```python
from build123d import *

# Parameters (mm, degrees)
SKETCH2_W           = 50
SKETCH2_H           = 52
BOSS_EXTRUDE1_DEPTH = 52
SKETCH3_W           = 50
SKETCH3_H           = 50
CUT_EXTRUDE1_DEPTH  = 50
CUT_EXTRUDE3_DEPTH  = 50
SKETCH5_R           = 2
CUT_EXTRUDE4_DEPTH  = 50
SKETCH7_W           = 52
SKETCH7_H           = 2
BOSS_EXTRUDE2_DEPTH = 5
SKETCH8_R           = 2.5
CUT_EXTRUDE6_DEPTH  = 5
SKETCH10_W          = 1
SKETCH10_H          = 2
CUT_EXTRUDE7_DEPTH  = 160
SKETCH11_W          = 48
SKETCH11_H          = 2
BOSS_EXTRUDE3_DEPTH = 3
SKETCH12_W          = 48
SKETCH12_H          = 2
BOSS_EXTRUDE4_DEPTH = 53
CUT_EXTRUDE9_DEPTH  = 53
FILLET1_R           = 24
FILLET2_R           = 24


with BuildPart() as part:
    # Sketch2 → Boss-Extrude1 (new body)
    with BuildSketch(Plane(origin=(0, 0, 0), x_dir=(1, 0, 0), z_dir=(0, 1, 0))):
        Rectangle(SKETCH2_W, SKETCH2_H)
    extrude(amount=BOSS_EXTRUDE1_DEPTH)

    # Sketch3 → Cut-Extrude1 (cut)
    with BuildSketch(Plane(origin=(0, 52, 0), x_dir=(1, 0, 0), z_dir=(0, 1, 0))):
        with Locations((0, -1)):
            Rectangle(SKETCH3_W, SKETCH3_H)
    extrude(amount=-CUT_EXTRUDE1_DEPTH, mode=Mode.SUBTRACT)

    # Sketch4 → Cut-Extrude3 (cut)
    with BuildSketch(Plane.XY.offset(-24)):
        with BuildLine():
            Line((-6.92820323, 18), (0, 18))
            Line((0, 18), (0, 24))
            ThreePointArc((0, 24), (-5, 29), (0, 34))
            Line((0, 34), (0, 40))
            Line((0, 40), (-6.92820323, 40))
            ThreePointArc((-6.92820323, 40), (-13, 29), (-6.92820323, 18))
        make_face()
        with BuildLine():
            Line((0, 24), (0, 18))
            Line((0, 18), (6.92820323, 18))
            ThreePointArc((6.92820323, 18), (13, 29), (6.92820323, 40))
            Line((6.92820323, 40), (0, 40))
            Line((0, 40), (0, 34))
            ThreePointArc((0, 34), (3.535533906, 32.535533906), (5, 29))
            ThreePointArc((5, 29), (3.535533906, 25.464466094), (0, 24))
        make_face()
    extrude(amount=-CUT_EXTRUDE3_DEPTH, mode=Mode.SUBTRACT)


with BuildPart() as body_2:
    # of the pieces the cut leaves, the one that is kept (cut_extrude3_keep)
    add(part.part.solids().sort_by_distance((25, 0, 26))[0])

    # Sketch5 → Cut-Extrude4 (cut)
    with BuildSketch(Plane.XY.offset(-24)):
        with Locations((12.55, 41.55)):
            Circle(SKETCH5_R)
        with Locations((-12.55, 41.55)):
            Circle(SKETCH5_R)
        with Locations((12.55, 16.45)):
            Circle(SKETCH5_R)
        with Locations((-12.55, 16.45)):
            Circle(SKETCH5_R)
    extrude(amount=-CUT_EXTRUDE4_DEPTH, mode=Mode.SUBTRACT)

    # Sketch7 → Boss-Extrude2 (add)
    with BuildSketch(Plane(origin=(25, 0, 0), x_dir=(0, 0, -1), z_dir=(1, 0, 0))):
        with Locations((0, 1)):
            Rectangle(SKETCH7_W, SKETCH7_H)
    boss_extrude2 = extrude(amount=BOSS_EXTRUDE2_DEPTH)

    # Mirror1: Boss-Extrude2 across plane
    add(boss_extrude2.mirror(Plane(origin=(0, 0, 0), x_dir=(0, 0, 1), z_dir=(1, 0, 0))))

    # Sketch8 → Cut-Extrude6 (cut)
    with BuildSketch(Plane(origin=(0, 2, 0), x_dir=(1, 0, 0), z_dir=(0, 1, 0))):
        with Locations(Location((-26.5, 14, 0), (0, 0, 270))):
            Circle(SKETCH8_R)
        with Locations(Location((-26.5, -16, 0), (0, 0, 270))):
            Circle(SKETCH8_R)
        with Locations(Location((26.5, 14, 0), (0, 0, 270))):
            Circle(SKETCH8_R)
        with Locations(Location((26.5, -16, 0), (0, 0, 270))):
            Circle(SKETCH8_R)
    extrude(amount=-CUT_EXTRUDE6_DEPTH, mode=Mode.SUBTRACT)

    # Sketch10 → Cut-Extrude7 (cut)
    with BuildSketch(Plane(origin=(0, 52, 0), x_dir=(1, 0, 0), z_dir=(0, 1, 0))):
        Polygon((25, 24), (24, 24), (-24, 24), (-25, 24), (-25, 26), (-30, 26), (-30, -26), (30, -26), (30, 26), (25, 26), align=None)
        with Locations((-24.5, 25)):
            Rectangle(SKETCH10_W, SKETCH10_H)
        with Locations((24.5, 25)):
            Rectangle(SKETCH10_W, SKETCH10_H)
    extrude(amount=-CUT_EXTRUDE7_DEPTH, mode=Mode.SUBTRACT)

    # Sketch11 → Boss-Extrude3 (add)
    with BuildSketch(Plane(origin=(0, 52, 0), x_dir=(1, 0, 0), z_dir=(0, 1, 0))):
        with Locations((0, 25)):
            Rectangle(SKETCH11_W, SKETCH11_H)
    extrude(amount=BOSS_EXTRUDE3_DEPTH)

    # Sketch12 → Boss-Extrude4 (add)
    with BuildSketch(Plane.XY.offset(-24)):
        with Locations((0, 1)):
            Rectangle(SKETCH12_W, SKETCH12_H)
    extrude(amount=BOSS_EXTRUDE4_DEPTH)

    # Sketch13 → Cut-Extrude9 (cut)
    with BuildSketch(Plane(origin=(0, 2, 0), x_dir=(1, 0, 0), z_dir=(0, 1, 0))):
        with BuildLine():
            Line((19, 14.5), (14, 14.5))
            ThreePointArc((14, 14.5), (12, 16.5), (14, 18.5))
            Line((14, 18.5), (19, 18.5))
            ThreePointArc((19, 18.5), (21, 16.5), (19, 14.5))
        make_face()
        with BuildLine():
            Line((-19, 14.5), (-14, 14.5))
            ThreePointArc((-14, 14.5), (-12, 16.5), (-14, 18.5))
            Line((-14, 18.5), (-19, 18.5))
            ThreePointArc((-19, 18.5), (-21, 16.5), (-19, 14.5))
        make_face()
        with BuildLine():
            Line((-19, -21.5), (-14, -21.5))
            ThreePointArc((-14, -21.5), (-12, -23.5), (-14, -25.5))
            Line((-14, -25.5), (-19, -25.5))
            ThreePointArc((-19, -25.5), (-21, -23.5), (-19, -21.5))
        make_face()
        with BuildLine():
            Line((19, -21.5), (14, -21.5))
            ThreePointArc((14, -21.5), (12, -23.5), (14, -25.5))
            Line((14, -25.5), (19, -25.5))
            ThreePointArc((19, -25.5), (21, -23.5), (19, -21.5))
        make_face()
    extrude(amount=-CUT_EXTRUDE9_DEPTH, mode=Mode.SUBTRACT)

    # Fillet1
    fillet1_edges = [body_2.edges().sort_by_distance(p)[0] for p in [
        (-24, 55, -25),
    ]]
    fillet(fillet1_edges, radius=FILLET1_R)

    # Fillet2
    fillet2_edges = [body_2.edges().sort_by_distance(p)[0] for p in [
        (24, 55, -25),
    ]]
    fillet(fillet2_edges, radius=FILLET2_R - 0.0001)  # a hair under: the kernel refuses the full size


solid = body_2.part
```
Source: CAD feature listing. Evaluate the final solid. Frame: model axes, mm. A direction names the side the tool comes from. Give positions to 0.01 mm unless a question says otherwise; leave off trailing zeros. Write each loop counter-clockwise with the first axis right and the second up, starting at its lowest first coordinate (ties: lowest second). Pieces come first, ordered by that corner, then holes. Notation, with made-up numbers: (65, -19.75) - (96, -19.75) arc R35 cw to (96, 16.25) - close; hole circle Ø6 at (-21, 38.5). An arc over 180 degrees is marked (long way). One line per item, written item: value. Start each with the question number.
Q1. Section query B-B, the plane y = 32.5. Return the cut outline in (x, z).
Q2. Set-up query: faces 1 (the face through (16.78, 48.16, -25.01)), 2 (the face through (0, 16, -24)), 3 (the face through (0, 18, -25)), 4 (the face through (-21, 1, 23.5)), 5 (the face through (0, 15, -26)). Return all of +Z, -Z, +X, -X, +Y, -Y with unobstructed straight access to the full face (end or side cutting, diameter ignored); none if empty.
Q3. Section query D-D, the plane x = 3. Return the cut outline in (y, z), then the cut area to 3 significant figures.
Q4. Draft query along Y for faces 6 (the face through (-16, 1, -18.5)), 7 (the face through (-13, 14.5, -25)), 8 (the face through (0, 2, 2)). Return one class per face: +Y half, -Y half, draft (parallel to the pull), parting line (faces both ways), or undercut.
Q5. Material intervals for probe 1 along Y at (x, z) = (12, -25); probe 2 along Z at (x, y) = (-2, 15); probe 3 along Y at (x, z) = (-6, 21), sorted ascending. Write a range as from..to.
Q6. First-contact query: pin 1 Ø1 at (x, z) = (-1, -25) entering from +Y; pin 2 Ø10 at (x, y) = (-2.5, 33.5) entering from +Z; pin 3 Ø4.5 at (x, y) = (12.55, 16.45) entering from +Z. Flat tips, straight axial feed; report the tip coordinate or a pass-through.
Q7. Section query A-A, the plane z = -16.5. Return the cut outline in (x, y).
Q8. Section query C-C, the plane y = 41.55. Return the cut outline in (x, z).
Answer:
1. outline: (-23.95, -26) - (-12.52, -26) - (-12.52, -24) - (-23.95, -24) - close; (12.52, -26) - (23.95, -26) - (23.95, -24) - (12.52, -24) - close
2. face 1: +Z, -Z, +X, +Y
2. face 2: +Z, +X, -X, +Y
2. face 3: +Z, -Z
2. face 4: +Y, -Y
2. face 5: -Z, +X, -X, +Y, -Y
3. outline: (0, -26) - (18, -26) - (18, -24) - (2, -24) - (2, 29) - (0, 29) - close; (40, -26) - (54.81, -26) - (54.81, -24) - (40, -24) - close
3. area: 172 mm2
4. face 6: draft
4. face 7: undercut
4. face 8: +Y half
5. probe 1: y = 0..14.53, 18.37..24, 34..39.63, 43.47..51.78
5. probe 2: z = -26..-24
5. probe 3: y = 0..2
6. pin 1: stops at y = 54.99
6. pin 2: passes through
6. pin 3: stops at z = -24
7. outline: (-24, 0) - (-21, 0) - (-21, 2) - (-24, 2) - close; (-12, 0) - (12, 0) - (12, 2) - (-12, 2) - close; (21, 0) - (24, 0) - (24, 2) - (21, 2) - close
8. outline: (-21.56, -26) - (-14.55, -26) - (-14.55, -24) - (-21.56, -24) - close; (-10.55, -26) - (10.55, -26) - (10.55, -24) - (-10.55, -24) - close; (14.55, -26) - (21.56, -26) - (21.56, -24) - (14.55, -24) - close
